from build123d import *

# Parameters (mm, degrees)
SKETCH119_W             = 2
SKETCH119_H             = 6
POCKET017_DEPTH         = 2
CHAMFER006_SIZE         = 0.35
CHAMFER007_SIZE         = 0.75
BODY020_PLACEMENT_ANGLE = 90
BODY021_PLACEMENT_ANGLE = 10
BODY024_PLACEMENT_ANGLE = 90


with BuildPart() as part:
    # Sketch119 → Revolution002 (revolve)
    with BuildSketch(Plane.XZ):
        with Locations((-1, 3)):
            Rectangle(SKETCH119_W, SKETCH119_H)
    revolve(axis=Axis((0, 0, 0), (0, 0, 1)))

    # Sketch124 (on Face3 of Revolution002) → Pocket017 (cut)
    with BuildSketch(Plane(origin=(0, 0, 6), x_dir=(-1, 0, 0), z_dir=(0, 0, 1))):
        Polygon((-0.625, -1.0825317547), (0.625, -1.0825317547), (1.25, 0), (0.625, 1.0825317547), (-0.625, 1.0825317547), (-1.25, 0), align=None)
    extrude(amount=-POCKET017_DEPTH, mode=Mode.SUBTRACT)

    # Chamfer006
    chamfer006_edges = [part.edges().sort_by_distance(p)[0] for p in [
        (2, 0, 6),
    ]]
    chamfer(chamfer006_edges, length=CHAMFER006_SIZE)

    # Chamfer007
    chamfer007_edges = [part.edges().sort_by_distance(p)[0] for p in [
        (2, 0, 0),
    ]]
    chamfer(chamfer007_edges, length=CHAMFER007_SIZE)


with BuildPart() as part_1:
    # Body020 placement: moved
    add(part.part.moved(Location((0, -3, 4))).rotate(Axis((0, -3, 4), (1, 0, 0)), BODY020_PLACEMENT_ANGLE))


with BuildPart() as part_2:
    # Clone001 placement: moved
    add(part_1.part.moved(Location((0, -1, 0))))


with BuildPart() as part_3:
    # Body021 placement: moved
    add(part_2.part.moved(Location((-0.1736481777, 0.984807753, 17))).rotate(Axis((-0.1736481777, 0.984807753, 17), (0, 0, 1)), BODY021_PLACEMENT_ANGLE))


with BuildPart() as part_4:
    # Clone003 placement: moved
    add(part_3.part.moved(Location((0.1736481777, -0.984807753, 0))))


with BuildPart() as part_5:
    # Body024 placement: moved
    add(part_4.part.moved(Location((-1, 0, 0))).rotate(Axis((-1, 0, 0), (0, 0, 1)), BODY024_PLACEMENT_ANGLE))


solid = part_5.part
The listing builds one solid part. Answer for the finished solid, in the listing's coordinates (mm). A direction names the side the tool comes from. Coordinates: 2 decimals unless noted, no trailing zeros. Write each question's results on one line, items separated by ' | '.
Item 1: Given P1, Ø1, axis at x = 5.5, z = 19.5, coming from the -Y side, flat-ended and moving along its own axis, determine where the tip first touches the part or whether it passes through.
Answer below:
P1: y = -0.63
Item 2: Consider probe 1 along Y at (x, z) = (8.5, 21.35); probe 2 along Z at (x, y) = (8.5, 0.35); probe 3 along Z at (x, y) = (3.5, 1.5). Determine where each line is inside the solid, lowest interval first. Write a range as [from, to].
Answer below:
probe 1: [-0.32, 0.61], [2.74, 3.37] | probe 2: [19.48, 22.52] | probe 3: [19.19, 22.81]
Item 3: Which of the six approach directions +Z, -Z, +X, -X, +Y, -Y give full straight-line access (tool end or side, diameter ignored) to faces 1 (the face through (8.039, 0.646, 21.549)), 2 (the face through (7.714, 2.493, 21.534))?
Answer below:
face 1: none | face 2: +X
Item 4: For a pull along Z with two mould halves and no side action, classify faces 3 (the face through (2.936, 0.712, 20.982)), 4 (the face through (7.715, 2.484, 20.451)), 5 (the face through (6.079, 1.513, 19.017)) as released by +Z, released by -Z, zero draft, split by the parting line, or undercut.
Answer below:
face 3: zero draft | face 4: undercut | face 5: split by the parting line
